```python
from build123d import *

# Parameters (mm, degrees)
SKETCH_1_W          = 15
SKETCH_1_H          = 10
EXTRUDE_1_DEPTH     = 30
SKETCH_2_W          = 12
SKETCH_2_H          = 7
CUT_EXTRUDE_1_DEPTH = 28.5
SKETCH_3_R          = 2.6
CUT_EXTRUDE_2_DEPTH = 33.5
SKETCH_4_R          = 1.6
CUT_EXTRUDE_3_DEPTH = 1.5


with BuildPart() as part:
    # 草图1 → 凸台-拉伸1 (new body)
    with BuildSketch(Plane(origin=(0, 0, 0), x_dir=(1, 0, 0), z_dir=(0, 1, 0))):
        Rectangle(SKETCH_1_W, SKETCH_1_H)
    extrude(amount=EXTRUDE_1_DEPTH)

    # 草图2 → 切除-拉伸1 (cut)
    with BuildSketch(Plane(origin=(0, 30, 0), x_dir=(1, 0, 0), z_dir=(0, 1, 0))):
        Rectangle(SKETCH_2_W, SKETCH_2_H)
    extrude(amount=-CUT_EXTRUDE_1_DEPTH, mode=Mode.SUBTRACT)

    # 草图3 → 切除-拉伸2 (cut, through all)
    with BuildSketch(Plane.XY.offset(5)):
        with Locations((0, 20)):
            Circle(SKETCH_3_R)
    extrude(amount=-CUT_EXTRUDE_2_DEPTH, mode=Mode.SUBTRACT)

    # 草图4 → 切除-拉伸3 (cut)
    with BuildSketch(Plane(origin=(0, 0, -5), x_dir=(-1, 0, 0), z_dir=(0, 0, -1))):
        with Locations((0, 6.25)):
            Circle(SKETCH_4_R)
    extrude(amount=-CUT_EXTRUDE_3_DEPTH, mode=Mode.SUBTRACT)


solid = part.part
```
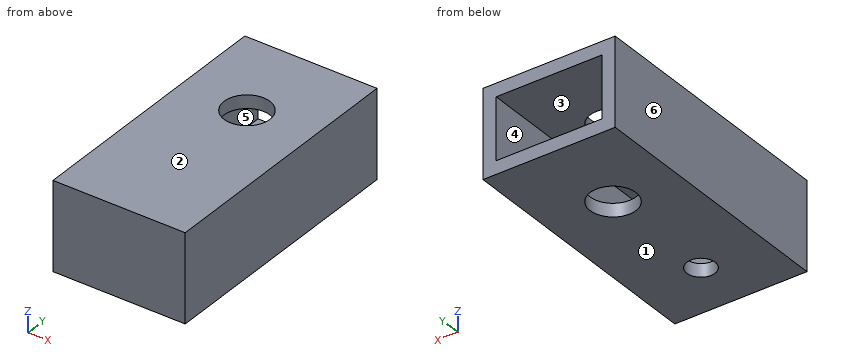
For this review, take the finished solid that the model builds, in its own axes (mm). Face numbers are marked on the shaded views. A direction names the side the tool comes from. Give positions to 0.01 mm unless a question says otherwise; leave off trailing zeros. Order: outer loops, then holes, each group sorted by start corner. A loop starts at its lowest first (then second) coordinate and runs counter-clockwise, first axis right, second up.
1) Take a section at A-A (x = 0). Give the boundary of the cut face in (y, z), then the cut area to 3 significant figures.
2) Take a section at C-C (y = 20). Give the boundary of the cut face in (x, z).
3) Take a section at B-B (y = 15.25). Give the boundary of the cut face in (x, z), then the cut area to 3 significant figures.
4) Wall thickness on line 1 (Y direction, x = 0, z = -3.9); line 2 (Z direction, x = -5, y = 13.75); line 3 (X direction, y = 10.5, z = -0.25): over which ranges is each line inside the solid? List them lowest first.
5) Take a section at D-D (x = 3). Give the boundary of the cut face in (y, z), then the cut area to 4 significant figures.
6) Insertion check: pin 1 (2 mm diameter, centred on x = -1.5, z = -1.5, fed in from +Y). The pin has a flat end and moves straight along its axis. Give the tip position at first contact, or say it passes through.
7) The part is to be moulded in two halves that separate along Z. For the marked faces 1, 2, 3 and 4, say which applies: released by +Z, released by -Z, zero draft, split by the parting line, or undercut.
8) For the marked faces 5 and 6, list the 3-axis set-ups (+Z, -Z, +X, -X, +Y, -Y) from which the entire face can be reached by the end or side of a thin tool; tool diameter is ignored.
Derived:
1. outline: (0, -5) - (4.65, -5) - (4.65, -3.5) - (1.5, -3.5) - (1.5, 3.5) - (17.4, 3.5) - (17.4, 5) - (0, 5) - close; (7.85, -5) - (17.4, -5) - (17.4, -3.5) - (7.85, -3.5) - close; (22.6, -5) - (30, -5) - (30, -3.5) - (22.6, -3.5) - close; (22.6, 3.5) - (30, 3.5) - (30, 5) - (22.6, 5) - close
1. area: 80.1 mm2
2. outline: (-7.5, -5) - (-2.6, -5) - (-2.6, -3.5) - (-6, -3.5) - (-6, 3.5) - (-2.6, 3.5) - (-2.6, 5) - (-7.5, 5) - close; (2.6, -5) - (7.5, -5) - (7.5, 5) - (2.6, 5) - (2.6, 3.5) - (6, 3.5) - (6, -3.5) - (2.6, -3.5) - close
3. outline: (-7.5, -5) - (7.5, -5) - (7.5, 5) - (-7.5, 5) - close; hole (-6, -3.5) - (6, -3.5) - (6, 3.5) - (-6, 3.5) - close
3. area: 66.0 mm2
4. line 1: y = 0 to 4.65, 7.85 to 17.4, 22.6 to 30
4. line 2: z = -5 to -3.5, 3.5 to 5
4. line 3: x = -7.5 to -6, 6 to 7.5
5. outline: (0, -5) - (30, -5) - (30, -3.5) - (1.5, -3.5) - (1.5, 3.5) - (30, 3.5) - (30, 5) - (0, 5) - close
5. area: 100.5 mm2
6. pin 1: stops at y = 1.5
7. face 1: released by -Z
7. face 2: released by +Z
7. face 3: undercut
7. face 4: undercut
8. face 5: +Y
8. face 6: +Z, -Z, -X, +Y, -Y
